```python
from build123d import *

# Parameters (mm, degrees)
SKETCH_1_W          = 12.5
SKETCH_1_H          = 4
EXTRUDE_1_DEPTH     = 4
FILLET_1_R          = 2
SKETCH_1_3_W        = 18.3
SKETCH_1_3_H        = 4
EXTRUDE_2_DEPTH     = 1
FILLET_2_R          = 2
SKETCH_2_R          = 0.75
CUT_EXTRUDE_1_DEPTH = 10.834759784
EXTRUDE_START       = -4
SKETCH_3_R          = 0.5
EXTRUDE_3_DEPTH     = 5.6
SKETCH_4_R          = 0.5
CUT_EXTRUDE_2_DEPTH = 0.1


with BuildPart() as part:
    # 草图1 → 凸台-拉伸1 (new body)
    with BuildSketch(Plane(origin=(0, 0, 0), x_dir=(1, 0, 0), z_dir=(0, 1, 0))):
        Rectangle(SKETCH_1_W, SKETCH_1_H)
    extrude(amount=EXTRUDE_1_DEPTH)

    # 圆角1
    fillet_1_edges = [part.edges().sort_by_distance(p)[0] for p in [
        (6.25, 2, -2),
        (6.25, 2, 2),
        (-6.25, 2, 2),
        (-6.25, 2, -2),
    ]]
    fillet(fillet_1_edges, radius=FILLET_1_R - 0.0001)  # a hair under: the kernel refuses the full size

    # 草图1<3> → 凸台-拉伸2 (add)
    with BuildSketch(Plane(origin=(0, 0, 0), x_dir=(1, 0, 0), z_dir=(0, 1, 0))):
        Rectangle(SKETCH_1_3_W, SKETCH_1_3_H)
    extrude(amount=EXTRUDE_2_DEPTH)

    # 圆角2
    fillet_2_edges = [part.edges().sort_by_distance(p)[0] for p in [
        (9.15, 0.5, 2),
        (9.15, 0.5, -2),
        (-9.15, 0.5, 2),
        (-9.15, 0.5, -2),
    ]]
    fillet(fillet_2_edges, radius=FILLET_2_R - 0.0001)  # a hair under: the kernel refuses the full size

    # 草图2 → 切除-拉伸1 (cut, through all)
    with BuildSketch(Plane(origin=(0, 1, 0), x_dir=(1, 0, 0), z_dir=(0, 1, 0))):
        with Locations(Location((-7.7, 0, 0), (0, 0, 270))):
            Circle(SKETCH_2_R)
        with Locations(Location((7.7, 0, 0), (0, 0, 270))):
            Circle(SKETCH_2_R)
    extrude(amount=-CUT_EXTRUDE_1_DEPTH, mode=Mode.SUBTRACT)

    # 草图3 → 凸台-拉伸3 (add)
    with BuildSketch(Plane.XZ.offset(EXTRUDE_START)):
        with Locations(Location((-1.27, 0, 0), (0, 0, 90))):
            Circle(SKETCH_3_R)
        with Locations(Location((1.27, 0, 0), (0, 0, 90))):
            Circle(SKETCH_3_R)
    extrude(amount=EXTRUDE_3_DEPTH)

    # 草图4 → 切除-拉伸2 (cut)
    with BuildSketch(Plane.XZ):
        with Locations(Location((0, 0, 0), (0, 0, 270))):
            Circle(SKETCH_4_R)
    extrude(amount=-CUT_EXTRUDE_2_DEPTH, mode=Mode.SUBTRACT)


solid = part.part
```
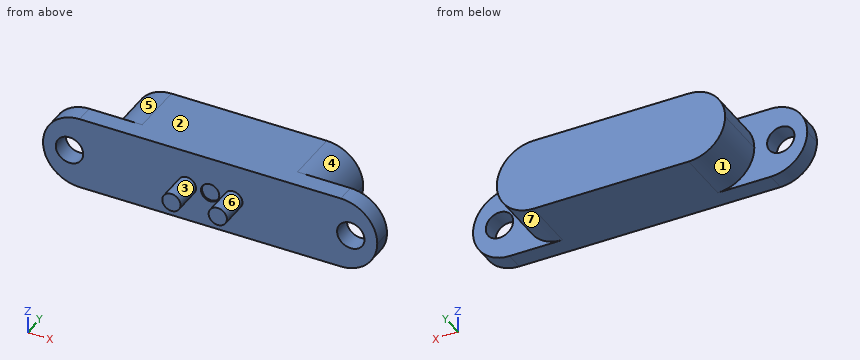
Model file for the job. Use its own axes, mm. Face numbers are marked on the shaded views. A direction names the side the tool comes from. Round coordinates to 2 decimals unless told otherwise and drop trailing zeros. Write each loop counter-clockwise with the first axis right and the second up, starting at its lowest first coordinate (ties: lowest second). Pieces come first, ordered by that corner, then holes. Notation, with made-up numbers: M -15,25.25 L 37,25.25 A21 ccw 37,31.25 Z; hole C 7.5,-26 d3. An arc over 180 degrees is marked long. Put each result on its own line as item: value.
Item 1: Probe L1, parallel to X at y = 0.35, z = 0; L2, parallel to X at y = 0.9, z = -0.4; L3, parallel to Y at x = 1, z = -0.8. List the from-to ranges inside material, lowest first. Write a range as from..to.
Responses:
L1: -9.15..-8.45, -6.95..6.95, 8.45..9.15
L2: -9.11..-8.33, -7.07..7.07, 8.33..9.11
L3: 0..4
Item 2: Flat gauge pins, fed straight in: P1, Ø1.7, axis at x = -7.7, z = 0, coming from the +Y side; P2, Ø1.5, axis at x = 0, z = 0.5, coming from the -Y side; P3, Ø2, axis at y = 3, z = 1.5, coming from the +X side. Where does each tip first touch, or does it go through?
Responses:
P1: y = 1
P2: y = 0
P3: x = 6.19
Item 3: Cut at C-C (z = -0.2). List the corners of the cut face in (x, y).
Responses:
outline: M -9.14,0 L -8.42,0 L -8.42,1 L -9.14,1 Z; M -6.98,0 L -1.73,0 L -1.73,-1.6 L -0.81,-1.6 L -0.81,0 L -0.46,0 L -0.46,0.1 L 0.46,0.1 L 0.46,0 L 0.81,0 L 0.81,-1.6 L 1.73,-1.6 L 1.73,0 L 6.98,0 L 6.98,1 L 6.24,1 L 6.24,4 L -6.24,4 L -6.24,1 L -6.98,1 Z; M 8.42,0 L 9.14,0 L 9.14,1 L 8.42,1 Z
Item 4: Cut at D-D (x = 8.25). List the corners of the cut face in (y, z), and give its area (3 significant figures).
Responses:
outline: M 0,-1.67 L 1,-1.67 L 1,-0.51 L 0,-0.51 Z; M 0,0.51 L 1,0.51 L 1,1.67 L 0,1.67 Z
area: 2.32 mm²
Item 5: Tool access for the marked faces 4, 5, 6 and 7: list every direction of +Z, -Z, +X, -X, +Y, -Y with a clear straight run to the whole face (end or side of a thin tool).
Responses:
face 4: +Z, +X, +Y
face 5: +Z, -X, +Y
face 6: -Y
face 7: -Z, +X, +Y
Item 6: Cut at B-B (y = -0.5). List the corners of the cut face in (x, z), and give its area (3 significant figures).
Responses:
outline: C -1.27,0 d1; C 1.27,0 d1
area: 1.57 mm²
Item 7: Cut at A-A (x = 0). List the corners of the cut face in (y, z).
Responses:
outline: M 0,-2 L 4,-2 L 4,2 L 0,2 L 0,0.5 L 0.1,0.5 L 0.1,-0.5 L 0,-0.5 Z
Item 8: Mould opens along X. For the marked faces 1, 2 and 3 say: +X half, -X half, draft (parallel to the pull), parting line (faces both ways), or undercut.
Responses:
face 1: -X half
face 2: draft
face 3: undercut
